Verification items for this drawing (mm, ordinates from the low corner). Give positions to 0.01 mm unless a question says otherwise; leave off trailing zeros. Loops run counter-clockwise (first coordinate to the right, second up) from the corner with the lowest first, then second, coordinate; pieces in that order, holes last. Notation, with made-up numbers: M 53.25,35.25 L 107.25,35.25 A29 cw 107.25,73.25 Z; hole C -5,71.5 d11. An arc over 180 degrees is marked long. Use one line per item in the form item = value.
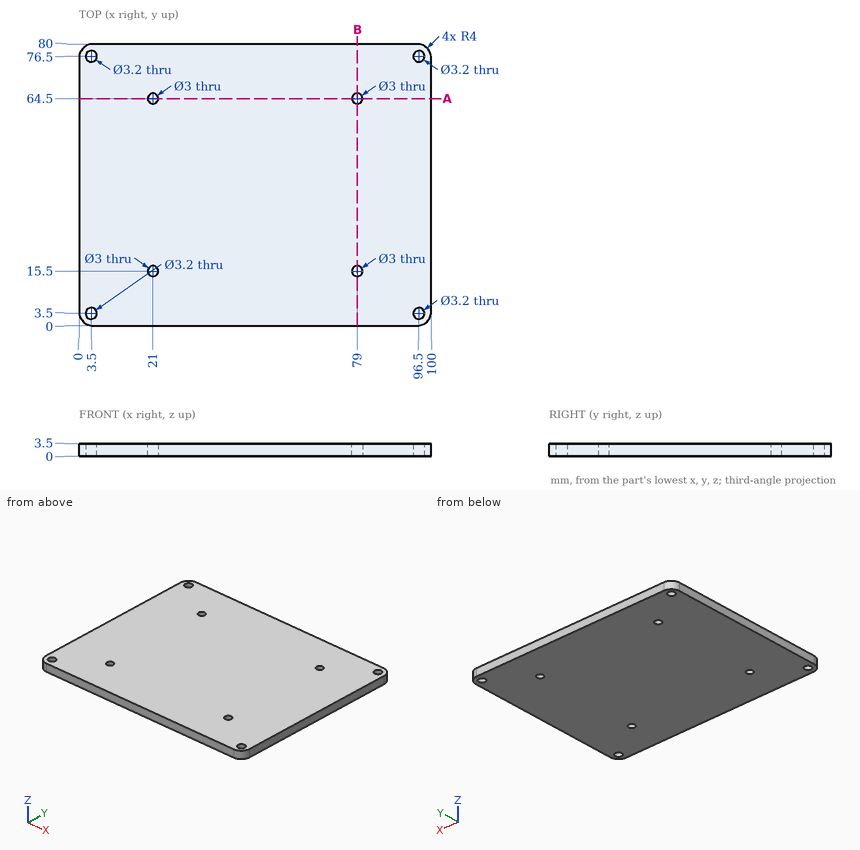
1) Section check B-B (x = 79). Record the cut outline in (y, z).
Evaluation:
outline = M 0,0 L 14,0 L 14,3.5 L 0,3.5 Z; M 17,0 L 63,0 L 63,3.5 L 17,3.5 Z; M 66,0 L 80,0 L 80,3.5 L 66,3.5 Z
2) Scan lines: line 1 (X direction, y = 64.5, z = 2.7); line 2 (X direction, y = 76.5, z = 1.6); line 3 (Y direction, x = 96.5, z = 1.9). Record each from-to range of solid material in increasing order.
Evaluation:
line_1 = 0 to 19.5, 22.5 to 77.5, 80.5 to 100
line_2 = 0.03 to 1.9, 5.1 to 94.9, 98.1 to 99.97
line_3 = 0.03 to 1.9, 5.1 to 74.9, 78.1 to 79.97
3) Section check A-A (y = 64.5). Record the cut outline in (x, z).
Evaluation:
outline = M 0,0 L 19.5,0 L 19.5,3.5 L 0,3.5 Z; M 22.5,0 L 77.5,0 L 77.5,3.5 L 22.5,3.5 Z; M 80.5,0 L 100,0 L 100,3.5 L 80.5,3.5 Z
